```python
from build123d import *

# Parameters (mm, degrees)
CUT_EXTRUDE1_DEPTH      = 157.294477939
CUT_EXTRUDE1_DEPTH_BACK = 157.294477939
CUT_EXTRUDE3_DEPTH      = 156.280037628
CUT_EXTRUDE3_DEPTH_BACK = 156.280037628
CUT_EXTRUDE4_DEPTH      = 155.479713623
CUT_EXTRUDE4_DEPTH_BACK = 155.479713623
SKETCH4_R               = 10


with BuildPart() as part:
    # Sketch1 → Revolve1 (revolve)
    with BuildSketch(Plane(origin=(0, 0, 0), x_dir=(0, 0, -1), z_dir=(1, 0, 0))):
        with BuildLine():
            Line((0, 31.048058087), (0, 0))
            Line((0, 0), (150, 0))
            Line((150, 0), (150, 19.53096248))
            Line((150, 19.53096248), (63.206041057, 19.53096248))
            ThreePointArc((63.206041057, 19.53096248), (60.040415158, 19.783081261), (56.954600633, 20.533081214))
            Line((56.954600633, 20.533081214), (28.045399367, 30.045939353))
            ThreePointArc((28.045399367, 30.045939353), (24.959584842, 30.795939306), (21.793958943, 31.048058087))
            Line((21.793958943, 31.048058087), (0, 31.048058087))
        make_face()
    revolve(axis=Axis((0, 0, -150), (0, 0, 1)))

    # Sketch2 → Cut-Extrude1 (cut, two sides: drawn at the far end of the back side and taken through both)
    with BuildSketch(Plane(origin=(0, 0, 0), x_dir=(0, 0, -1), z_dir=(1, 0, 0)).offset(-CUT_EXTRUDE1_DEPTH_BACK)):
        with BuildLine():
            Line((0, 20), (0, -20))
            Line((0, -20), (23.903263743, -20))
            ThreePointArc((23.903263743, -20), (27.730098067, -19.238795325), (30.974331555, -17.071067812))
            Line((30.974331555, -17.071067812), (39.071067812, -8.974331555))
            ThreePointArc((39.071067812, -8.974331555), (41.238795325, -5.730098067), (42, -1.903263743))
            Line((42, -1.903263743), (42, 1.903263743))
            ThreePointArc((42, 1.903263743), (41.238795325, 5.730098067), (39.071067812, 8.974331555))
            Line((39.071067812, 8.974331555), (30.974331555, 17.071067812))
            ThreePointArc((30.974331555, 17.071067812), (27.730098067, 19.238795325), (23.903263743, 20))
            Line((23.903263743, 20), (0, 20))
        make_face()
    extrude(amount=CUT_EXTRUDE1_DEPTH + CUT_EXTRUDE1_DEPTH_BACK, mode=Mode.SUBTRACT)

    # Sketch3 → Cut-Extrude3 (cut, two sides: drawn at the far end of the back side and taken through both)
    with BuildSketch(Plane(origin=(0, 0, 0), x_dir=(1, 0, 0), z_dir=(0, 1, 0)).offset(-CUT_EXTRUDE3_DEPTH_BACK)):
        with BuildLine():
            ThreePointArc((0, 0), (-14.142135624, 5.857864376), (-20, 20))
            Line((-20, 20), (-20, 58.900056316))
            Line((-20, 58.900056316), (-33.967415872, 58.900056316))
            Line((-33.967415872, 58.900056316), (-33.967415872, 0))
            Line((-33.967415872, 0), (0, 0))
        make_face()
        with BuildLine():
            ThreePointArc((20, 20), (14.142135624, 5.857864376), (0, 0))
            Line((0, 0), (30.596408204, 0))
            Line((30.596408204, 0), (30.596408204, 58.900056316))
            Line((30.596408204, 58.900056316), (20, 58.900056316))
            Line((20, 58.900056316), (20, 20))
        make_face()
    extrude(amount=CUT_EXTRUDE3_DEPTH + CUT_EXTRUDE3_DEPTH_BACK, mode=Mode.SUBTRACT)

    # Sketch4 → Cut-Extrude4 (cut, two sides: drawn at the far end of the back side and taken through both)
    with BuildSketch(Plane(origin=(0, 0, 0), x_dir=(1, 0, 0), z_dir=(0, 1, 0)).offset(-CUT_EXTRUDE4_DEPTH_BACK)):
        with Locations(Location((0, 20, 0), (0, 0, 169.665425663))):
            Circle(SKETCH4_R)
    extrude(amount=CUT_EXTRUDE4_DEPTH + CUT_EXTRUDE4_DEPTH_BACK, mode=Mode.SUBTRACT)


solid = part.part
```
CAD build for the part. Positions are in the model's coordinates, mm. A direction names the side the tool comes from. Give positions to 0.01 mm unless a question says otherwise; leave off trailing zeros. Order: outer loops, then holes, each group sorted by start corner. A loop starts at its lowest first (then second) coordinate and runs counter-clockwise, first axis right, second up. Notation, with made-up numbers: M 11.25,81.25 L 23.25,81.25 A23 cw 23.25,93.25 Z; hole C 67.5,-2.5 d2. An arc over 180 degrees is marked long. Put each result on its own line as item: value. Start each with the question number.
(1) Flat gauge pins, fed straight in: pin 1 Ø8 at (x, z) = (1.5, -86.5) entering from -Y; pin 2 Ø1.5 at (x, z) = (-7, -116.5) entering from -Y; pin 3 Ø7 at (x, z) = (5, -15.5) entering from -Y. Where does each tip first touch, or does it go through?
(2) Mould opens along Y. For faces 1 (the cylindrical face through (-0.304, -31.047, -8.323)), 2 (the flat face through (-20, -0.1, -42.2)), 3 (the cylindrical face through (-0.28, 17.336, -30.7)) say: +Y half, -Y half, draft (parallel to the pull), parting line (faces both ways), or undercut.
(3) Drill centre lines: line 1 along X through (y, z) = (-23.25, -20); line 2 along X through (y, z) = (25, -20); line 3 along Z through (x, y) = (0, -2). Where is each one in solid material? Low to high.
(4) Which spindle directions (+Z, -Z, +X, -X, +Y, -Y) get a long thin tool onto all of the face, cutting with end or side? Do faces 4 (the flat face through (0, 0, -42)), 5 (the conical face through (-0.457, -24.295, -45.51)), 6 (the cylindrical face through (7.48, 18.04, -106)). Say none if no direction does.
(5) Saw through at B-B, the plane z = -65. Write the cut outline in (x, y).
(6) Saw through at A-A, the plane y = 0. Write the cut outline in (x, z), then the cut area to 3 significant figures.
Check result:
1. pin 1: stops at y = -19.53
1. pin 2: stops at y = -18.5
1. pin 3: stops at y = -30.39
2. face 1: -Y half
2. face 2: draft
2. face 3: undercut
3. line 1: x = -20 to -10, 10 to 20
3. line 2: x = -18.41 to -10, 10 to 18.41
3. line 3: z = -150 to -42
4. face 4: +Z, +X, -X
4. face 5: -Z, -Y
4. face 6: -Z
5. outline: C 0,0 d39.06
6. outline: M -20,-58.9 A20 cw -19.53,-63.21 L -19.53,-150 L 19.53,-150 L 19.53,-63.21 A20 cw 20,-58.9 L 20,-42 L -20,-42 Z
6. area: 4,240 mm2
